from build123d import *

# Parameters (mm, degrees)
SKETCH1_R           = 1.499950003
SKETCH1_R_2         = 1.49995001
SKETCH1_W           = 3.0001
SKETCH1_H           = 8
BOSS_EXTRUDE1_DEPTH = 3.175


with BuildPart() as part:
    # Sketch1 → Boss-Extrude1 (new body)
    with BuildSketch(Plane(origin=(0, 0, 0), x_dir=(1, 0, 0), z_dir=(0, 1, 0))):
        with BuildLine():
            Line((-15.7526, 12.89915), (15.1125, 12.89915))
            add(Edge.make_bspline(
                [(15.1125, 12.89915), (17.575103024, 13.12464748), (19.77450252, 11.294353024), (20, 8.83175)],
                knots=[0.111111111, 0.111111111, 0.111111111, 0.111111111, 0.222222222, 0.222222222, 0.222222222, 0.222222222], degree=3))
            Line((20, 8.83175), (20, -8.83175))
            add(Edge.make_bspline(
                [(20, -8.83175), (19.77450252, -11.294353024), (17.575103024, -13.12464748), (15.1125, -12.89915)],
                knots=[0.333333333, 0.333333333, 0.333333333, 0.333333333, 0.444444444, 0.444444444, 0.444444444, 0.444444444], degree=3))
            Line((15.1125, -12.89915), (-15.7526, -12.89915))
            add(Edge.make_bspline(
                [(-15.7526, -12.89915), (-18.039200664, -12.948650664), (-19.950499336, -11.118350664), (-20, -8.83175)],
                knots=[0.555555556, 0.555555556, 0.555555556, 0.555555556, 0.666666667, 0.666666667, 0.666666667, 0.666666667], degree=3))
            Line((-20, -8.83175), (-20, 8.83175))
            add(Edge.make_bspline(
                [(-20, 8.83175), (-19.950499336, 11.118350664), (-18.039200664, 12.948650664), (-15.7526, 12.89915)],
                knots=[0.777777778, 0.777777778, 0.777777778, 0.777777778, 1, 1, 1, 1], degree=3))
        make_face()
        with Locations(Location((-4.06191002, 10.083599991, 0), (0, 0, 270))):
            Circle(SKETCH1_R, mode=Mode.SUBTRACT)
        with Locations(Location((-4.06191002, -9.71635, 0), (0, 0, 270))):
            Circle(SKETCH1_R_2, mode=Mode.SUBTRACT)
        Polygon((-15.5612, 5.98375), (7.4388, 5.98375), (7.4388, -6.41625), (-15.5612, -6.41625), (-15.5612, -2.71635), (-17.5613, -2.71635), (-17.5613, 2.28365), (-15.5612, 2.28365), align=None, mode=Mode.SUBTRACT)
        with Locations((15.87435, -0.21635)):
            Rectangle(SKETCH1_W, SKETCH1_H, mode=Mode.SUBTRACT)
    extrude(amount=BOSS_EXTRUDE1_DEPTH)


solid = part.part
Design review of the part built by this model. Coordinates are the model's own, in mm. A direction names the side the tool comes from. Coordinates: 2 decimals unless noted, no trailing zeros. Loops run counter-clockwise (first coordinate to the right, second up) from the corner with the lowest first, then second, coordinate; pieces in that order, holes last. Notation, with made-up numbers: (39, 10.25) - (45, 10.25) arc R21 ccw to (45, 19.25) - close; hole circle Ø11 at (54, 66). An arc over 180 degrees is marked (long way). Use CSV: the item, a comma, the result in double quotes. Start each with the question number.
1. Add section B-B on z = -0.25. Give the boundary of the cut face in (x, y) (3 decimals).
2. Add section D-D on y = 1.1. Count the separate pieces of the cut face and the enclosed holes in it, plus the area to 3 significant figures.
3. Clearance check with flat-ended pins moving along their axes: pin 1 (12 mm diameter, centred on x = 3.5, z = 5, fed in from +Y) (3 decimals); pin 2 (0.9 mm diameter, centred on x = 16.5, y = 1.5, fed in from +Z); pin 3 (1 mm diameter, centred on x = -16, y = 2.5, fed in from -Z). State where each tip first meets the part, or that it passes through.
4. Add section C-C on x = -5. Give the boundary of the cut face in (y, z) (3 decimals).
5. Add section A-A on x = 2.5. Give the boundary of the cut face in (y, z) (3 decimals), plus the area to 3 significant figures.
6. For faces 1 (the flat face through (-20, 2, 0)), 2 (the flat face through (14.374, 2, 0)), list the 3-axis set-ups (+Z, -Z, +X, -X, +Y, -Y) from which the entire face can be reached by the end or side of a thin tool; tool diameter is ignored.
7. Mouldability with a two-part tool opening along Z and no side actions: class faces 3 (the flat face through (0, 2, 12.899)), 4 (the flat face through (9, 3.175, 0)), 5 (the cylindrical face through (-4.975, 1.565, 8.526)), 6 (the flat face through (-1, 2, -12.899)) as released by +Z, released by -Z, zero draft, split by the parting line, or undercut.
8. To check wall thickness, follow probe 1 along X at (y, z) = (0.5, -3); probe 2 along X at (y, z) = (2.3, 0.5); probe 3 along Z at (x, y) = (-11, 2.1). State the ranges of each line that lie inside material, in increasing order.
Resolved:
1,outline,"(-20, 0) - (-17.561, 0) - (-17.561, 3.175) - (-20, 3.175) - close; (7.439, 0) - (14.374, 0) - (14.374, 3.175) - (7.439, 3.175) - close; (17.374, 0) - (20, 0) - (20, 3.175) - (17.374, 3.175) - close"
2,separate pieces,"1"
2,enclosed holes,"4"
2,area,"683 mm2"
3,pin 1,"y = 3.175"
3,pin 2,"z = 12.89"
3,pin 3,"z = -12.9"
4,outline,"(0, -12.899) - (3.175, -12.899) - (3.175, -11.254) - (0, -11.254) - close; (0, -8.913) - (3.175, -8.913) - (3.175, -5.984) - (0, -5.984) - close; (0, 6.416) - (3.175, 6.416) - (3.175, 8.546) - (0, 8.546) - close; (0, 10.887) - (3.175, 10.887) - (3.175, 12.899) - (0, 12.899) - close"
5,outline,"(0, -12.899) - (3.175, -12.899) - (3.175, -5.984) - (0, -5.984) - close; (0, 6.416) - (3.175, 6.416) - (3.175, 12.899) - (0, 12.899) - close"
5,area,"42.5 mm2"
6,face 1,"+Z, -Z, -X, +Y, -Y"
6,face 2,"+Y, -Y"
7,face 3,"released by +Z"
7,face 4,"zero draft"
7,face 5,"undercut"
7,face 6,"released by -Z"
8,probe 1,"-20 to -15.56, 7.44 to 14.37, 17.37 to 20"
8,probe 2,"-20 to -17.56, 7.44 to 14.37, 17.37 to 20"
8,probe 3,"-12.9 to -5.98, 6.42 to 12.9"
